```python
from build123d import *

# Parameters (mm, degrees)
SKETCH1_W           = 30
SKETCH1_H           = 30
BOSS_EXTRUDE1_DEPTH = 15.5
FILLET1_R           = 2
SKETCH2_R           = 14
CUT_EXTRUDE1_DEPTH  = 21
SKETCH3_R           = 1.6
CUT_EXTRUDE2_DEPTH  = 15
CUT_EXTRUDE3_DEPTH  = 37.949289574
SKETCH5_R           = 1.6
CUT_EXTRUDE4_DEPTH  = 46.169126725
CUT_EXTRUDE5_DEPTH  = 2.95
SKETCH7_R           = 2.85
CUT_EXTRUDE6_DEPTH  = 2.95
BOSS_EXTRUDE2_START = -18.5
BOSS_EXTRUDE2_DEPTH = 7
SKETCH9_R           = 1.6
CUT_EXTRUDE7_DEPTH  = 43.320326157


with BuildPart() as part:
    # Sketch1 → Boss-Extrude1 (new, symmetric)
    with BuildSketch(Plane(origin=(0, 0, 0), x_dir=(0, 0, -1), z_dir=(1, 0, 0))):
        with Locations((-15, 0)):
            Rectangle(SKETCH1_W, SKETCH1_H)
    extrude(amount=BOSS_EXTRUDE1_DEPTH, both=True)

    # Fillet1
    fillet1_edges = [part.edges().sort_by_distance(p)[0] for p in [
        (0, -15, 0),
        (0, -15, 30),
        (0, 15, 30),
        (0, 15, 0),
    ]]
    fillet(fillet1_edges, radius=FILLET1_R)

    # Sketch2 → Cut-Extrude1 (cut)
    with BuildSketch(Plane(origin=(15.5, 0, 0), x_dir=(0, 0, -1), z_dir=(1, 0, 0))):
        with Locations((-15, 0)):
            Circle(SKETCH2_R)
    extrude(amount=-CUT_EXTRUDE1_DEPTH, mode=Mode.SUBTRACT)

    # Sketch3 → Cut-Extrude2 (cut)
    with BuildSketch(Plane(origin=(15.5, 0, 0), x_dir=(0, 0, -1), z_dir=(1, 0, 0))):
        with Locations((-27, 12)):
            Circle(SKETCH3_R)
        with Locations((-3, 12)):
            Circle(SKETCH3_R)
        with Locations((-3, -12)):
            Circle(SKETCH3_R)
        with Locations((-27, -12)):
            Circle(SKETCH3_R)
    extrude(amount=-CUT_EXTRUDE2_DEPTH, mode=Mode.SUBTRACT)

    # Sketch4 → Cut-Extrude3 (cut, through all)
    with BuildSketch(Plane.XY.offset(30)):
        with BuildLine():
            Line((-6.25, 9), (-15.5, 9))
            Line((-15.5, 9), (-15.5, -9))
            Line((-15.5, -9), (-6.25, -9))
            ThreePointArc((-6.25, -9), (11.75, 0), (-6.25, 9))
        make_face()
    extrude(amount=-CUT_EXTRUDE3_DEPTH, mode=Mode.SUBTRACT)

    # Sketch5 → Cut-Extrude4 (cut, through all)
    with BuildSketch(Plane(origin=(0, 15, 0), x_dir=(1, 0, 0), z_dir=(0, 1, 0))):
        with Locations(Location((-12, -5, 0), (0, 0, 270))):
            Circle(SKETCH5_R)
        with Locations(Location((-12, -25, 0), (0, 0, 270))):
            Circle(SKETCH5_R)
    extrude(amount=-CUT_EXTRUDE4_DEPTH, mode=Mode.SUBTRACT)

    # Sketch6 → Cut-Extrude5 (cut)
    with BuildSketch(Plane(origin=(0, 15, 0), x_dir=(1, 0, 0), z_dir=(0, 1, 0))):
        Polygon((-10.387287493, -7.7933), (-8.774574986, -5), (-10.387287493, -2.2067), (-13.612712507, -2.2067), (-15.225425014, -5), (-13.612712507, -7.7933), align=None)
        Polygon((-8.774574986, -25), (-10.387287493, -22.2067), (-13.612712507, -22.2067), (-15.225425014, -25), (-13.612712507, -27.7933), (-10.387287493, -27.7933), align=None)
    extrude(amount=-CUT_EXTRUDE5_DEPTH, mode=Mode.SUBTRACT)

    # Sketch7 → Cut-Extrude6 (cut)
    with BuildSketch(Plane.XZ.offset(15)):
        with Locations(Location((-12, 25, 0), (0, 0, 270))):
            Circle(SKETCH7_R)
        with Locations(Location((-12, 5, 0), (0, 0, 270))):
            Circle(SKETCH7_R)
    extrude(amount=-CUT_EXTRUDE6_DEPTH, mode=Mode.SUBTRACT)

    # Sketch8 → Boss-Extrude2 (add)
    with BuildSketch(Plane(origin=(15.5, 0, 0), x_dir=(0, 0, -1), z_dir=(1, 0, 0)).offset(BOSS_EXTRUDE2_START)):
        with BuildLine():
            Line((-29.6463, -14.135647969), (-29.6463, -19))
            ThreePointArc((-29.6463, -19), (-27.334438807, -22.361651144), (-23.368134214, -21.405707385))
            Line((-23.368134214, -21.405707385), (-17.6141, -15))
            Line((-17.6141, -15), (-28, -15))
            ThreePointArc((-28, -15), (-28.929705346, -14.770776092), (-29.6463, -14.135647969))
        make_face()
    extrude(amount=BOSS_EXTRUDE2_DEPTH)

    # Sketch9 → Cut-Extrude7 (cut, through all)
    with BuildSketch(Plane(origin=(4, 0, 0), x_dir=(0, 0, -1), z_dir=(1, 0, 0))):
        with Locations((-26.5, -19.5)):
            Circle(SKETCH9_R)
    extrude(amount=-CUT_EXTRUDE7_DEPTH, mode=Mode.SUBTRACT)


solid = part.part
```
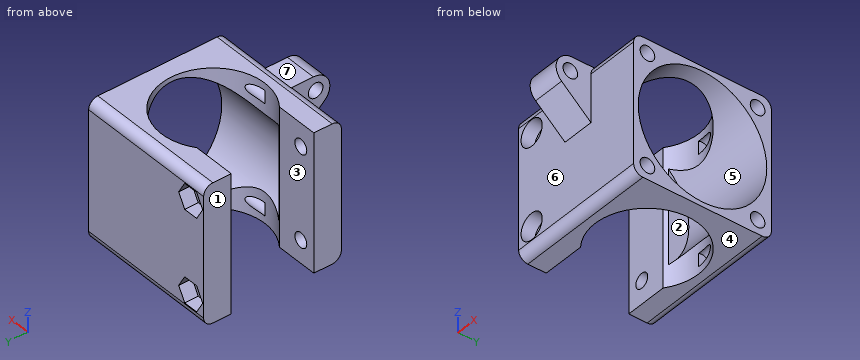
For this review, take the finished solid that the model builds, in its own axes (mm). Face numbers are marked on the shaded views. A direction names the side the tool comes from. Round coordinates to 2 decimals unless told otherwise and drop trailing zeros. Write each loop counter-clockwise with the first axis right and the second up, starting at its lowest first coordinate (ties: lowest second). Pieces come first, ordered by that corner, then holes. Notation, with made-up numbers: M 39.25,-0.75 L 53.25,-0.75 A32 ccw 53.25,33.25 Z; hole C -36,64.25 d5. An arc over 180 degrees is marked long. One line per item, written item: value. Start each with the question number.
(1) Wall thickness on line 1 (Z direction, x = 10.25, y = 12); line 2 (Z direction, x = -11, y = 13); line 3 (X direction, y = -13.75, z = 5): over which ranges is each line inside the solid? List them lowest first.
(2) We need section A-A (z = 15). Give the boundary of the cut face in (x, y).
(3) The part is to be moulded in two halves that separate along Z. For the marked faces 4, 5, 6 and 7, say which applies: released by +Z, released by -Z, zero draft, split by the parting line, or undercut.
(4) Machinability: for the marked faces 1, 2 and 3, which of the approach directions +Z, -Z, +X, -X, +Y, -Y give a long, thin tool a straight path to every point of the face, cutting with its end or side? Answer none if there is none.
(5) We need section B-B (x = -8). Give the boundary of the cut face in (y, z), and give its area (3 significant figures).
(6) Insertion check: pin 1 (8 mm diameter, centred on x = 2.5, z = 17.5, fed in from -Y); pin 2 (1.7 mm diameter, centred on x = -11, z = 4, fed in from -Y); pin 3 (3 mm diameter, centred on x = -5.5, z = 23, fed in from -Y). Each pin has a flat end and moves straight along its axis. Give the tip position at first contact, or say it passes through.
(7) We need section C-C (x = 5.5). Give the boundary of the cut face in (y, z), and give its area (3 significant figures).
(8) We need section D-D (y = 2). Give the boundary of the cut face in (x, z).
Result:
1. line 1: 0 to 1.4, 4.6 to 7.79, 22.21 to 25.4, 28.6 to 30
1. line 2: 0 to 2.21, 7.79 to 22.21, 27.79 to 30
1. line 3: -15.5 to -14.85, -9.15 to 15.5
2. outline: M -15.5,-15 L 15.5,-15 L 15.5,-14 L -5.5,-14 L -5.5,-9.52 A11.25 cw -6.25,-9 L -15.5,-9 Z; M -15.5,9 L -6.25,9 A11.25 cw -5.5,9.52 L -5.5,14 L 15.5,14 L 15.5,15 L -15.5,15 Z
3. face 4: released by -Z
3. face 5: undercut
3. face 6: zero draft
3. face 7: released by +Z
4. face 1: +Z, -Z, -X, +Y, -Y
4. face 2: +X
4. face 3: +Z, -Z, -X
5. outline: M -15,2 A2 ccw -13,0 L -9,0 L -9,30 L -13,30 A2 ccw -15,28 Z; M 9,0 L 13,0 A2 ccw 15,2 L 15,28 A2 ccw 13,30 L 9,30 Z
5. area: 357 mm²
6. pin 1: y = -19.33
6. pin 2: y = -12.05
6. pin 3: y = -15
7. outline: M -15,2 A2 ccw -13,0 L -10.08,0 L -10.08,5.28 A14 cw -10.08,24.72 L -10.08,30 L -13,30 A2 ccw -15,28 Z; M 10.08,0 L 13,0 A2 ccw 15,2 L 15,28 A2 ccw 13,30 L 10.08,30 L 10.08,24.72 A14 cw 10.08,5.28 Z; hole C -12,3 d3.2; hole C -12,27 d3.2; hole C 12,3 d3.2; hole C 12,27 d3.2
7. area: 155 mm²
8. outline: M 11.57,0 L 15.5,0 L 15.5,1.14 L 11.57,1.14 Z; M 11.57,28.86 L 15.5,28.86 L 15.5,30 L 11.57,30 Z
